from build123d import *

# Parameters (mm, degrees)
BOSS_EXTRUDE1_DEPTH = 10
SKETCH3_W           = 208.746083537
SKETCH3_H           = 274.535725978
CUT_EXTRUDE1_DEPTH  = 399.651564654


with BuildPart() as part:
    # Sketch2 → Boss-Extrude1 (new body)
    with BuildSketch(Plane.XY.offset(-4)):
        with BuildLine():
            Line((-300, 17.25), (-9.906933746, 17.25))
            ThreePointArc((-9.906933746, 17.25), (-7.67705834, 17.349645471), (-5.464958693, 17.647787546))
            ThreePointArc((-5.464958693, 17.647787546), (173.262167791, 29.246699007), (349.996014284, 0.211065854))
            ThreePointArc((349.996014284, 0.211065854), (359.352395656, -4.784442191), (365.795573071, -13.209549776))
            Line((365.795573071, -13.209549776), (400.384507401, -86.847766013))
            ThreePointArc((400.384507401, -86.847766013), (400.778842945, -87.899120346), (401, -89))
            ThreePointArc((401, -89), (399.447287587, -94.279668904), (394.557793346, -96.805270939))
            ThreePointArc((394.557793346, -96.805270939), (214.863177419, -108.403215094), (35, -117))
            Line((35, -117), (-30.25, -117))
            Line((-30.25, -117), (-293.242078622, -117))
            ThreePointArc((-293.242078622, -117), (-293.197036902, -109.999972274), (-293.25, -103))
            ThreePointArc((-293.25, -103), (-297.900702689, -41.860509444), (-310, 18.25))
            ThreePointArc((-310, 18.25), (-305.024937811, 17.500621894), (-300, 17.25))
        make_face()
        with BuildLine():
            Line((-300, 15.25), (-9.906933746, 15.25))
            ThreePointArc((-9.906933746, 15.25), (-7.498668308, 15.357617109), (-5.109600689, 15.67961055))
            ThreePointArc((-5.109600689, 15.67961055), (173.164177958, 27.249100951), (349.449732641, -1.712882265))
            ThreePointArc((349.449732641, -1.712882265), (358.057603503, -6.308749667), (363.985326724, -14.059848645))
            Line((363.985326724, -14.059848645), (398.574261055, -87.698064882))
            ThreePointArc((398.574261055, -87.698064882), (398.855929301, -88.449032263), (399.013898626, -89.235374873))
            ThreePointArc((399.013898626, -89.235374873), (397.904818331, -93.006566947), (394.412322444, -94.8105684))
            ThreePointArc((394.412322444, -94.8105684), (214.770700526, -106.405257008), (34.960579781, -115))
            Line((34.960579781, -115), (-30.25, -115))
            Line((-30.25, -115), (-291.219119939, -115))
            ThreePointArc((-291.219119939, -115), (-291.198633765, -108.985341109), (-291.250212173, -102.970868486))
            ThreePointArc((-291.250212173, -102.970868486), (-295.709152828, -43.127202467), (-307.277212671, 15.756806448))
            ThreePointArc((-307.277212671, 15.756806448), (-303.647419534, 15.376854871), (-300, 15.25))
        make_face(mode=Mode.SUBTRACT)
    extrude(amount=BOSS_EXTRUDE1_DEPTH)

    # Sketch3 → Cut-Extrude1 (cut, through all)
    with BuildSketch(Plane(origin=(20, 0, 0), x_dir=(0, 0, -1), z_dir=(1, 0, 0))):
        with Locations((3.946589657, -49.091759287)):
            Rectangle(SKETCH3_W, SKETCH3_H)
    extrude(amount=-CUT_EXTRUDE1_DEPTH, mode=Mode.SUBTRACT)


solid = part.part
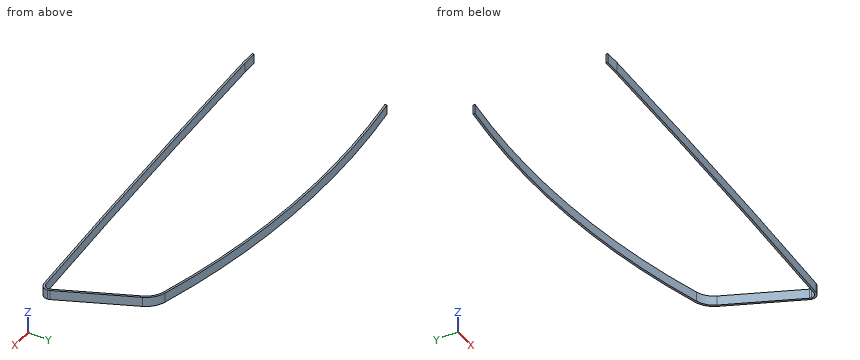
Geometry check sheet. Reference: the model listing, model coordinates, mm. Give positions to 0.01 mm unless a question says otherwise; leave off trailing zeros. Loops run counter-clockwise (first coordinate to the right, second up) from the corner with the lowest first, then second, coordinate; pieces in that order, holes last.
(1) Thickness scan on L1, parallel to Y at x = 186.5, z = -0.25; L2, parallel to Y at x = 357, z = 2.75; L3, parallel to X at y = -66, z = 1.25. Record the ranges inside material, lowest first.
From the geometry:
L1: y = -109.96 to -107.96, 26.48 to 28.49
L2: y = -99.48 to -97.47, -5.46 to -3.01
L3: x = 388.38 to 390.59
(2) Section check B-B on z = -1. Record the cut outline in (x, y), then the cut area to 3 significant figures.
From the geometry:
outline: (20, -117) - (35, -117) arc R10787.05 ccw to (394.56, -96.81) arc R7 ccw to (400.38, -86.85) - (365.8, -13.21) arc R25 ccw to (350, 0.21) arc R788.48 ccw to (20, 21.82) - (20, 19.79) arc R786.48 cw to (349.45, -1.71) arc R23 cw to (363.99, -14.06) - (398.57, -87.7) arc R5 cw to (394.41, -94.81) arc R10785.05 cw to (34.96, -115) - (20, -115) - close
area: 1,640 mm2
(3) Section check A-A on x = 128. Record the cut outline in (y, z), then the cut area to 3 significant figures.
From the geometry:
outline: (-112.93, -4) - (-110.93, -4) - (-110.93, 6) - (-112.93, 6) - close; (28.17, -4) - (30.17, -4) - (30.17, 6) - (28.17, 6) - close
area: 40.0 mm2
(4) Section check C-C on x = 74. Record the cut outline in (y, z).
From the geometry:
outline: (-115.39, -4) - (-113.39, -4) - (-113.39, 6) - (-115.39, 6) - close; (25.85, -4) - (27.86, -4) - (27.86, 6) - (25.85, 6) - close
(5) Depth check by flat-ended pin: pin 1 Ø4 at (x, z) = (270, -1) entering from +Y; pin 2 Ø1.5 at (y, z) = (-77.5, 0.5) entering from +X; pin 3 Ø1 at (y, z) = (-28, 1) entering from +X. Enter the tip coordinate at first touch or a pass-through.
From the geometry:
pin 1: stops at y = 18.83
pin 2: stops at x = 396.35
pin 3: stops at x = 372.98
(6) Section check D-D on y = -64.5. Record the cut outline in (x, z), then the cut area to 3 significant figures.
From the geometry:
outline: (387.68, -4) - (389.89, -4) - (389.89, 6) - (387.68, 6) - close
area: 22.1 mm2
